Source: CAD feature listing. Evaluate the final solid. Frame: model axes, mm. Round coordinates to 2 decimals unless told otherwise and drop trailing zeros. Loops run counter-clockwise (first coordinate to the right, second up) from the corner with the lowest first, then second, coordinate; pieces in that order, holes last. Notation, with made-up numbers: (42.25, 47.5) -> (94.25, 47.5) arc R20 ccw to (94.25, 83.5) -> close; hole circle Ø1 at (64, 59.5). An arc over 180 degrees is marked (long way). Return JSON: item names as keys, results as strings. Group by question number.
```python
from build123d import *

# Parameters (mm, degrees)
SKETCH1_W                                     = 69.85
SKETCH1_H                                     = 44.45
BOSS_EXTRUDE1_DEPTH                           = 4.7498
CSK_FOR_1_4_FLAT_HEAD_MACHINE_SCREW1_AT_COUNT = 2
CSK_FOR_1_4_FLAT_HEAD_MACHINE_SCREW1_AT_PITCH = 38.1
FILLET1_R                                     = 0.127


with BuildPart() as part:
    # Sketch1 → Boss-Extrude1 (new body)
    with BuildSketch(Plane.XY):
        with Locations((0, 22.225)):
            Rectangle(SKETCH1_W, SKETCH1_H)
    extrude(amount=BOSS_EXTRUDE1_DEPTH)

    # Sketch4 → CSK for 1/4 Flat Head Machine Screw1 (revolve, cut)
    with BuildSketch(Plane(origin=(19.05, 25.4, 4.7498), x_dir=(0, -1, 0), z_dir=(1, 0, 0))):
        Polygon((0, 0), (0, 4.7498), (3.3782, 4.7498), (3.3782, 3.520932584), (6.4389, 0), align=None)
    csk_for_1_4_flat_head_machine_screw1 = revolve(axis=Axis((19.05, 25.4, 11.0998), (0, 0, -1)), mode=Mode.SUBTRACT)

    # CSK for 1/4 Flat Head Machine Screw1 at: CSK for 1/4 Flat Head Machine Screw1 ×2
    with Locations(*[(-i * CSK_FOR_1_4_FLAT_HEAD_MACHINE_SCREW1_AT_PITCH, 0, 0) for i in range(1, CSK_FOR_1_4_FLAT_HEAD_MACHINE_SCREW1_AT_COUNT)]):
        add(csk_for_1_4_flat_head_machine_screw1, mode=Mode.SUBTRACT)

    # Fillet1
    fillet1_edges = [part.edges().sort_by_distance(p)[0] for p in [
        (0, 44.45, 4.7498),
        (34.925, 22.225, 4.7498),
        (0, 0, 4.7498),
        (34.925, 22.225, 0),
        (0, 44.45, 0),
        (-34.925, 22.225, 0),
        (0, 0, 0),
        (34.925, 0, 2.3749),
        (34.925, 44.45, 2.3749),
        (-34.925, 44.45, 2.3749),
        (-34.925, 0, 2.3749),
        (-34.925, 22.225, 4.7498),
    ]]
    fillet(fillet1_edges, radius=FILLET1_R)


solid = part.part
```
(1) Ray query, line 1 (X direction, y = 25.4, z = 0.5) (3 decimals); line 2 (Y direction, x = 19.05, z = 0.85); line 3 (X direction, y = 26, z = 3.7) (3 decimals). Return the intervals inside material, ascending.
(2) Cut plane A-A (y = 25.4). Return loops of the section in (x, z) (3 decimals), and give its area (3 significant figures).
(3) Cut plane B-B (x = -19.05). Return loops of the section in (y, z), and give its area (3 significant figures).
(4) Pin query (flat end, axial travel): pin 1 (5.5 mm diameter, centred on x = 19.05, y = 25.4, fed in from -Z). Return the tip coordinate at first contact, or that it passes through.
(5) Cut plane C-C (z = 2.5). Return loops of the section in (x, y) (3 decimals), and give its area (3 significant figures).
(6) Mould query, pull axis Y, two halves, no side actions, for faces 1 (the face through (0, 23, 0)), 2 (the face through (0, 0, 2)), 3 (the face through (22.535, 26.174, 1.449)). Classes: released by +Y, released by -Y, zero draft, split by the parting line, or undercut.
Answers follow:
{
 "1": {"line 1": "-34.925 to -22.428, -15.672 to 15.672, 22.428 to 34.925", "line 2": "0 to 22.02, 28.78 to 44.45", "line 3": "-34.925 to -24.544, -13.556 to 13.556, 24.544 to 34.925"},
 "2": {"outline": "(-34.925, 0.127) arc R0.127 ccw to (-34.798, 0) -> (-22.428, 0) -> (-22.428, 1.229) -> (-25.489, 4.75) -> (-34.798, 4.75) arc R0.127 ccw to (-34.925, 4.623) -> close; (-15.672, 0) -> (15.672, 0) -> (15.672, 1.229) -> (12.611, 4.75) -> (-12.611, 4.75) -> (-15.672, 1.229) -> close; (22.428, 0) -> (34.798, 0) arc R0.127 ccw to (34.925, 0.127) -> (34.925, 4.623) arc R0.127 ccw to (34.798, 4.75) -> (25.489, 4.75) -> (22.428, 1.229) -> close", "area": "246 mm^2"},
 "3": {"outline": "(0, 0.13) arc R0.13 ccw to (0.13, 0) -> (22.02, 0) -> (22.02, 1.23) -> (18.96, 4.75) -> (0.13, 4.75) arc R0.13 ccw to (0, 4.62) -> close; (28.78, 0) -> (44.32, 0) arc R0.13 ccw to (44.45, 0.13) -> (44.45, 4.62) arc R0.13 ccw to (44.32, 4.75) -> (31.84, 4.75) -> (28.78, 1.23) -> close", "area": "168 mm^2"},
 "4": {"pin 1": "through"},
 "5": {"outline": "(-34.925, 0.127) arc R0.127 ccw to (-34.798, 0) -> (34.798, 0) arc R0.127 ccw to (34.925, 0.127) -> (34.925, 44.323) arc R0.127 ccw to (34.798, 44.45) -> (-34.798, 44.45) arc R0.127 ccw to (-34.925, 44.323) -> close; hole circle Ø8.966 at (-19.05, 25.4); hole circle Ø8.966 at (19.05, 25.4)", "area": "2,980 mm^2"},
 "6": {"face 1": "zero draft", "face 2": "released by -Y", "face 3": "undercut"}
}
